Here's how the part is built. I have some questions about the finished solid (model axes, mm). Face numbers are marked on the shaded views. Coordinates: 2 decimals unless noted, no trailing zeros. Loops run counter-clockwise (first coordinate to the right, second up) from the corner with the lowest first, then second, coordinate; pieces in that order, holes last. Notation, with made-up numbers: (2.5, 65) - (24.5, 65) arc R19 cw to (24.5, 85) - close; hole circle Ø10 at (38, -5.75). An arc over 180 degrees is marked (long way). Use a Markdown table: item, result.
```python
from build123d import *


with BuildPart() as part:
    # Sketch1 → Revolve1 (revolve)
    with BuildSketch(Plane.XY):
        with BuildLine():
            Line((13, 8.5), (10.25, 8.5))
            Line((10.25, 8.5), (31.5, 63.5))
            Line((31.5, 63.5), (31.313440373, 63.572079856))
            Line((31.313440373, 63.572079856), (10.035591338, 8.5))
            Line((10.035591338, 8.5), (0, 8.5))
            Line((0, 8.5), (0, -13))
            ThreePointArc((0, -13), (9.192388155, -9.192388155), (13, 0))
            Line((13, 0), (13, 8.5))
        make_face()
    revolve(axis=Axis((0, -13, 0), (0, 1, 0)))


solid = part.part
```
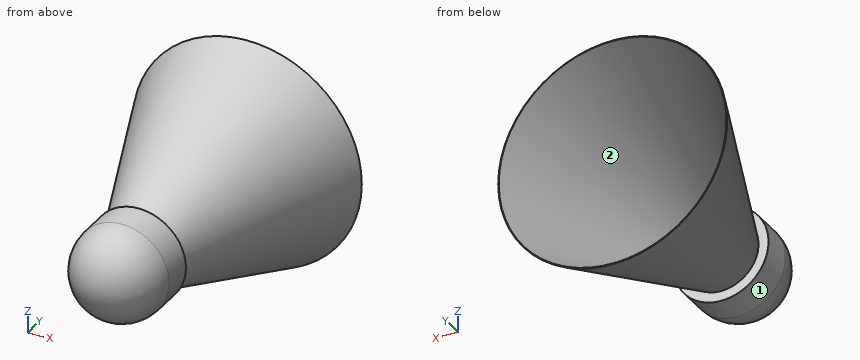
Q1. Will these pins go through, and if not, where does the flat tip stop? P1, Ø1.5, axis at x = 23, y = 47, coming from the -Z side; P2, Ø3, axis at x = 1.5, z = -11, coming from the -Y side; P3, Ø5, axis at y = 13.5, z = -2, coming from the +X side; P4, Ø12, axis at x = 22.5, z = 16.5, coming from the +Y side.
Check values:
| item | result |
|---|---|
| P1 | z = -11.8 |
| P2 | y = -8.76 |
| P3 | x = 13.04 |
| P4 | y = 63.57 |
Q2. I want a section at B-B, the plane x = 0. Write out the boundary of the cut face in (y, z).
Check values:
| item | result |
|---|---|
| outline | (0, -13) - (8.5, -13) - (8.5, -10.25) - (63.5, -31.5) - (63.57, -31.31) - (8.5, -10.04) - (8.5, 10.04) - (63.57, 31.31) - (63.5, 31.5) - (8.5, 10.25) - (8.5, 13) - (0, 13) arc R13 ccw to start |
Q3. I want a section at A-A, the plane z = 0. Write out the boundary of the cut face in (x, y).
Check values:
| item | result |
|---|---|
| outline | (-31.5, 63.5) - (-10.25, 8.5) - (-13, 8.5) - (-13, 0) arc R13 ccw to (13, 0) - (13, 8.5) - (10.25, 8.5) - (31.5, 63.5) - (31.31, 63.57) - (10.04, 8.5) - (-10.04, 8.5) - (-31.31, 63.57) - close |
Q4. I want a section at C-C, the plane y = 42.5. Write out the boundary of the cut face in (x, z), then the cut area to 3 significant figures.
Check values:
| item | result |
|---|---|
| outline | circle Ø46.77 at (0, 0); hole circle Ø46.34 at (0, 0) |
| area | 31.4 mm^2 |
Q5. If we mould it in two halves opening along X, with no side actions, what happens to the marked faces 1 and 2? For each: pulls with the +X half, pulls with the -X half, needs draft (parallel to the pull), parting line crosses it, or undercut.
Check values:
| item | result |
|---|---|
| face 1 | parting line crosses it |
| face 2 | undercut |
Q6. I want a section at D-D, the plane y = -4. Write out the boundary of the cut face in (x, z), then the cut area to 3 significant figures.
Check values:
| item | result |
|---|---|
| outline | circle Ø24.74 at (0, 0) |
| area | 481 mm^2 |
Q7. Please list where these lines run through material, in increasing order: L1, parallel to X at y = 59.5, z = 22; L2, parallel to X at y = 18.5, z = 4; L3, parallel to Z at x = 14, y = 32.5. Write a range as from..to.
Check values:
| item | result |
|---|---|
| L1 | -20.33..-20.01, 20.01..20.33 |
| L2 | -13.53..-13.31, 13.31..13.53 |
| L3 | -13.61..-13.3, 13.3..13.61 |
